Work out the finished part from the listing and answer in its coordinate system (mm). Face numbers are marked on the shaded views. A direction names the side the tool comes from. Round coordinates to 2 decimals unless told otherwise and drop trailing zeros. Loops run counter-clockwise (first coordinate to the right, second up) from the corner with the lowest first, then second, coordinate; pieces in that order, holes last. Notation, with made-up numbers: (52.25, 13) -> (104.25, 13) arc R29 cw to (104.25, 46) -> close; hole circle Ø4 at (-1.5, 41.25). An arc over 180 degrees is marked (long way). Write item = value, one per line. Start each with the question number.
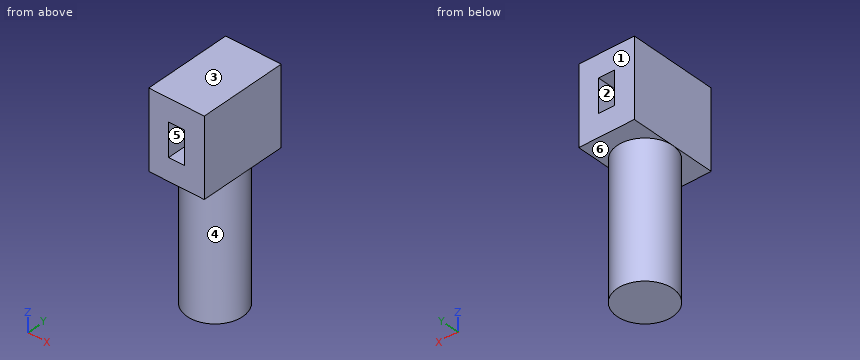
Autodesk Inventor part; units mm, degrees
ref_plane "YZ Plane" through (0, 0, 0) normal (1, 0, 0) x (0, 1, 0)
ref_plane "XZ Plane" through (0, 0, 0) normal (0, 1, 0) x (-1, 0, 0)
ref_plane "XY Plane" through (0, 0, 0) normal (0, 0, 1) x (1, 0, 0)
sketch "Sketch1" plane through (0, 0, 0) normal (0, 0, 1) x (1, 0, 0)
  circle A0 centre (0, 0) radius 25
  dimension "d0" = 50
extrude "Extrusion1" add sketch "Sketch1" along normal blind 120
sketch "Sketch5" plane through (0, 0, 120) normal (0, 0, 1) x (1, 0, 0)
  line L0 (-25, -40) -> (25, -40)
  line L1 (25, -40) -> (25, 40)
  line L2 (25, 40) -> (-25, 40)
  line L3 (-25, 40) -> (-25, -40)
  line L4 (-25, -40) -> (25, 40) construction
  line L5 (25, -40) -> (-25, 40) construction
  point P0 (0, 0)
  dimension "d18" = 50
  dimension "d19" = 80
extrude "Extrusion4" add sketch "Sketch5" along normal blind 70
sketch "Sketch6" plane through (-25, 40, 120) normal (0, 1, 0) x (1, 0, 0)
  point P0 (25, 120)
sketch "Sketch7" plane through (-25, 40, 120) normal (0, 1, 0) x (1, 0, 0)
  line L0 (0, 0) -> (50, 0)
  line L1 (0, -70) -> (50, -70)
  line L2 (50, 0) -> (0, -70)
  line L3 (32.1175, -49.918) -> (17.8825, -49.918)
  line L4 (17.8825, -49.918) -> (17.8825, -20.082)
  line L5 (17.8825, -20.082) -> (32.1175, -20.082)
  line L6 (32.1175, -20.082) -> (32.1175, -49.918)
  line L7 (32.1175, -49.918) -> (17.8825, -20.082) construction
  line L8 (17.8825, -49.918) -> (32.1175, -20.082) construction
  point P0 (25, 120)
  point P1 (25, -35)
  dimension "d22" = 14.235
  dimension "d23" = 29.836
extrude "Extrusion5" cut sketch "Sketch7" against normal through all
properties part number "武士刀夾具"
Item 1: Section D-D (x = -9.5) is taken. Determine the outline of the cut face in (y, z).
Item 2: Find the intervals of material crossed by line 1 along Z through (x, y) = (6, 36.5); line 2 along X through (y, z) = (-29, 152); line 3 along Z through (x, y) = (-16, -36.5), in increasing order. Write a range as [from, to].
Item 3: Section B-B (z = 157) is taken. Determine the outline of the cut face in (x, y).
Item 4: The mould has two halves that part along Z. Classify the marked faces 1, 2 and 3: pulls with the +Z half, pulls with the -Z half, needs draft (parallel to the pull), parting line crosses it, or undercut.
Item 5: Section A-A (x = 0) is taken. Determine the outline of the cut face in (y, z), then the cut area to 3 significant figures.
Item 6: Flat-ended cylindrical pins translate along their axes: pin 1 (3 mm diameter, centred on x = 3.5, z = 107.5, fed in from -Y); pin 2 (2 mm diameter, centred on x = -11.5, z = 111.5, fed in from -Y); pin 3 (12 mm diameter, centred on x = 17.5, z = 57.5, fed in from +Y). Find the tip coordinate at first contact, or state that the pin passes through.
Item 7: A tool of negligible diameter and unlimited length cuts with its end or side. For the marked faces 4, 5 and 6, from which of +Z, -Z, +X, -X, +Y, -Y can it reach the whole face along a straight path? Write none if from no direction.
Item 8: Section C-C (y = -34.5) is taken. Determine the outline of the cut face in (x, z), then the cut area to 3 significant figures.
Worked answers:
q1.outline = (-40, 120) -> (-23.12, 120) -> (-23.12, 0) -> (23.12, 0) -> (23.12, 120) -> (40, 120) -> (40, 190) -> (-40, 190) -> close
q2.line_1 = [120, 140.08], [169.92, 190]
q2.line_2 = [-25, -7.12], [7.12, 25]
q2.line_3 = [120, 190]
q3.outline = (-25, -40) -> (-7.12, -40) -> (-7.12, 40) -> (-25, 40) -> close; (7.12, -40) -> (25, -40) -> (25, 40) -> (7.12, 40) -> close
q4.face_1 = needs draft
q4.face_2 = undercut
q4.face_3 = pulls with the +Z half
q5.outline = (-40, 120) -> (-25, 120) -> (-25, 0) -> (25, 0) -> (25, 120) -> (40, 120) -> (40, 140.08) -> (-40, 140.08) -> close; (-40, 169.92) -> (40, 169.92) -> (40, 190) -> (-40, 190) -> close
q5.area = 9,210 mm2
q6.pin_1 = -24.92
q6.pin_2 = -22.69
q6.pin_3 = 22.2
q7.face_4 = -Z
q7.face_5 = +Y, -Y
q7.face_6 = -Z, +Y
q8.outline = (-25, 120) -> (25, 120) -> (25, 190) -> (-25, 190) -> close; hole (-7.12, 140.08) -> (7.12, 140.08) -> (7.12, 169.92) -> (-7.12, 169.92) -> close
q8.area = 3,080 mm2
